Part model, mm, in its own coordinate system. Face numbers are marked on the shaded views. A direction names the side the tool comes from. Coordinates: 2 decimals unless noted, no trailing zeros. Order: outer loops, then holes, each group sorted by start corner. A loop starts at its lowest first (then second) coordinate and runs counter-clockwise, first axis right, second up.
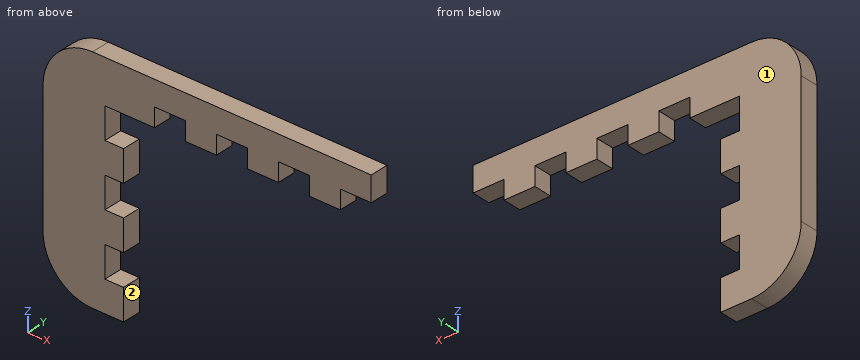
```python
from build123d import *

# Parameters (mm, degrees)
SKETCH1_W           = 48
SKETCH1_H           = 37
BOSS_EXTRUDE1_DEPTH = 3
SKETCH3_W           = 35
SKETCH3_H           = 30
CUT_EXTRUDE1_DEPTH  = 3
SKETCH5_W           = 5
SKETCH5_H           = 3
CUT_EXTRUDE2_DEPTH  = 3
SKETCH4_W           = 5
SKETCH4_H           = 3
CUT_EXTRUDE3_DEPTH  = 3
SKETCH6_W           = 4
SKETCH6_H           = 3
BOSS_EXTRUDE2_DEPTH = 5
FILLET2_R           = 8


with BuildPart() as part:
    # Sketch1 → Boss-Extrude1 (new body)
    with BuildSketch(Plane(origin=(0, 0, 0), x_dir=(1, 0, 0), z_dir=(0, 1, 0))):
        Rectangle(SKETCH1_W, SKETCH1_H)
    extrude(amount=BOSS_EXTRUDE1_DEPTH)

    # Sketch3 → Cut-Extrude1 (cut)
    with BuildSketch(Plane(origin=(0, 3, 0), x_dir=(1, 0, 0), z_dir=(0, 1, 0))):
        with Locations((6.5, 3.5)):
            Rectangle(SKETCH3_W, SKETCH3_H)
    extrude(amount=-CUT_EXTRUDE1_DEPTH, mode=Mode.SUBTRACT)

    # Sketch5 → Cut-Extrude2 (cut)
    with BuildSketch(Plane(origin=(-11, 0, 0), x_dir=(0, 0, -1), z_dir=(1, 0, 0))):
        with Locations((11, 1.5)):
            Rectangle(SKETCH5_W, SKETCH5_H)
        with Locations((1, 1.5)):
            Rectangle(SKETCH5_W, SKETCH5_H)
        with Locations((-9, 1.5)):
            Rectangle(SKETCH5_W, SKETCH5_H)
    extrude(amount=-CUT_EXTRUDE2_DEPTH, mode=Mode.SUBTRACT)

    # Sketch4 → Cut-Extrude3 (cut)
    with BuildSketch(Plane(origin=(0, 0, 11.5), x_dir=(-1, 0, 0), z_dir=(0, 0, -1))):
        with Locations((-16.5, 1.5)):
            Rectangle(SKETCH4_W, SKETCH4_H)
        with Locations((-6.5, 1.5)):
            Rectangle(SKETCH4_W, SKETCH4_H)
        with Locations((3.5, 1.5)):
            Rectangle(SKETCH4_W, SKETCH4_H)
    extrude(amount=-CUT_EXTRUDE3_DEPTH, mode=Mode.SUBTRACT)

    # Sketch6 → Boss-Extrude2 (add)
    with BuildSketch(Plane(origin=(24, 0, 0), x_dir=(0, 0, -1), z_dir=(1, 0, 0))):
        with Locations((-16.5, 1.5)):
            Rectangle(SKETCH6_W, SKETCH6_H)
    extrude(amount=BOSS_EXTRUDE2_DEPTH)

    # Fillet2
    fillet2_edges = [part.edges().sort_by_distance(p)[0] for p in [
        (-24, 1.5, 18.5),
        (-24, 1.5, -18.5),
    ]]
    fillet(fillet2_edges, radius=FILLET2_R)


solid = part.part
```
(1) Slice it at A-A, the plane x = -12. Give the cut face in (y, z).
(2) Probe line 1 (Z direction, x = -12.5, y = 2.45); line 2 (X direction, y = 2.4, z = 12.5); line 3 (Z direction, x = 5, y = 1.5). List the from-to ranges inside material, lowest first.
(3) Drop flat-ended pins along their axis: pin 1 (1 mm diameter, centred on y = 0.5, z = 13.5, fed in from -X); pin 2 (1.5 mm diameter, centred on x = 26.5, y = 2, fed in from -Z); pin 3 (0.9 mm diameter, centred on y = 1, z = -5, fed in from +X). Give the stop position or say it passes through.
(4) Slice it at B-B, the plane z = 12.5. Give the cut face in (x, y), then the cut area to 3 significant figures.
(5) Tool access for the marked faces 1 and 2: list every direction of +Z, -Z, +X, -X, +Y, -Y with a clear straight run to the whole face (end or side of a thin tool).
(6) Slice it at D-D, the plane z = 0. Give the cut face in (x, y).
Here are the results:
1. outline: (0, -18.5) - (3, -18.5) - (3, -13.5) - (0, -13.5) - close; (0, -8.5) - (3, -8.5) - (3, -3.5) - (0, -3.5) - close; (0, 1.5) - (3, 1.5) - (3, 6.5) - (0, 6.5) - close; (0, 11.5) - (3, 11.5) - (3, 18.5) - (0, 18.5) - close
2. line 1: z = -18.5 to -13.5, -8.5 to -3.5, 1.5 to 6.5, 11.5 to 18.5
2. line 2: x = -23.75 to -6, -1 to 4, 9 to 14, 19 to 24
2. line 3: z = 14.5 to 18.5
3. pin 1: stops at x = -23.6
3. pin 2: stops at z = 14.5
3. pin 3: stops at x = -11
4. outline: (-23.75, 0) - (-6, 0) - (-6, 3) - (-23.75, 3) - close; (-1, 0) - (4, 0) - (4, 3) - (-1, 3) - close; (9, 0) - (14, 0) - (14, 3) - (9, 3) - close; (19, 0) - (24, 0) - (24, 3) - (19, 3) - close
4. area: 98.2 mm2
5. face 1: +Z, -Z, +X, -X, +Y
5. face 2: -Z, +X, +Y, -Y
6. outline: (-24, 0) - (-14, 0) - (-14, 3) - (-24, 3) - close
